from build123d import *

# Parameters (mm, degrees)
SKETCH1_W                 = 60
SKETCH1_H                 = 50
BOSS_EXTRUDE1_DEPTH       = 40
SKETCH2_W                 = 70
SKETCH2_H                 = 70
BOSS_EXTRUDE2_DEPTH       = 1.5
SHELL1_START              = -28
SHELL1_OUTLINE_W          = 46
SHELL1_OUTLINE_H          = 39.5
SHELL1_DEPTH              = 56
F_3_0MM_DOWEL_HOLE2_D     = 3
F_3_0MM_DOWEL_HOLE2_DEPTH = 41.499
FILLET1_R                 = 2
CUT_EXTRUDE2_DEPTH        = 84.200060096
CUT_EXTRUDE2_DEPTH_BACK   = 84.200060096
SKETCH8_W                 = 56
SKETCH8_H                 = 39.5
SKETCH9_W                 = 1.5
SKETCH9_H                 = 70
CUT_EXTRUDE3_DEPTH        = 2


# Read off the part's stored shape, not the designer's step: Shell1
with BuildPart() as part:
    # Sketch1 → Boss-Extrude1 (new body)
    with BuildSketch(Plane.XY):
        Rectangle(SKETCH1_W, SKETCH1_H)
    extrude(amount=BOSS_EXTRUDE1_DEPTH)

    # Sketch2 → Boss-Extrude2 (add)
    with BuildSketch(Plane.XY.offset(40)):
        with Locations((-5, 0)):
            Rectangle(SKETCH2_W, SKETCH2_H)
    extrude(amount=BOSS_EXTRUDE2_DEPTH)

    # Shell1 outline → Shell1 (cut)
    with BuildSketch(Plane.YZ.offset(SHELL1_START)):
        with Locations((0, 21.75)):
            Rectangle(SHELL1_OUTLINE_W, SHELL1_OUTLINE_H)
    extrude(amount=SHELL1_DEPTH, mode=Mode.SUBTRACT)

    # Ø3.0mm Dowel Hole2
    with Locations(Plane(origin=(-311.781139065, -231.688044449, 0), x_dir=(-1, 0, 0), z_dir=(0, 0, -1))):
        with Locations((-327.471139065, 246.969744449), (-297.471139065, 246.969744449), (-297.471139065, 214.569744449), (-327.471139065, 214.569744449)):
            Hole(F_3_0MM_DOWEL_HOLE2_D / 2, depth=F_3_0MM_DOWEL_HOLE2_DEPTH)

    # Fillet1
    fillet1_edges = [part.edges().sort_by_distance(p)[0] for p in [
        (0, -25, 0),
        (-30, 0, 0),
        (0, 25, 0),
        (30, 0, 0),
        (30, -25, 20),
        (-30, -25, 20),
        (-30, 25, 20),
        (30, 25, 20),
    ]]
    fillet(fillet1_edges, radius=FILLET1_R)

    # Sketch8 → Cut-Extrude2 (cut, two sides: drawn at the far end of the back side and taken through both)
    with BuildSketch(Plane.XZ.offset(25).offset(-CUT_EXTRUDE2_DEPTH_BACK)):
        with Locations((0, 21.75)):
            Rectangle(SKETCH8_W, SKETCH8_H)
    extrude(amount=CUT_EXTRUDE2_DEPTH + CUT_EXTRUDE2_DEPTH_BACK, mode=Mode.SUBTRACT)

    # Sketch9 → Cut-Extrude3 (cut)
    with BuildSketch(Plane(origin=(30, 0, 0), x_dir=(0, 0, -1), z_dir=(1, 0, 0))):
        with Locations((-40.75, 0)):
            Rectangle(SKETCH9_W, SKETCH9_H)
    extrude(amount=-CUT_EXTRUDE3_DEPTH, mode=Mode.SUBTRACT)


solid = part.part
CAD build for the part. Positions are in the model's coordinates, mm. A direction names the side the tool comes from. Round coordinates to 2 decimals unless told otherwise and drop trailing zeros. Write each loop counter-clockwise with the first axis right and the second up, starting at its lowest first coordinate (ties: lowest second). Pieces come first, ordered by that corner, then holes.
(1) Slice it at C-C, the plane y = 21. Write the cut outline in (x, z), and give its area (3 significant figures).
(2) Slice it at A-A, the plane x = 15.69. Write the cut outline in (y, z).
(3) Drop flat-ended pins along their axis: P1, Ø3, axis at x = 8.5, y = 12, coming from the -Z side; P2, Ø10, axis at y = 25.5, z = 12.5, coming from the -X side; P3, Ø10, axis at x = -19, z = 5.5, coming from the -Y side; P4, Ø2.5, axis at x = -14.31, y = -17.12, coming from the +Z side. Give the stop position or say it passes through.
(4) Probe line 1 along X through (y, z) = (-6.5, 20.5); line 2 along Y through (x, z) = (15.69, 1.4); line 3 along Z through (x, y) = (-36, 22.5). List the from-to ranges inside material, lowest first.
(5) 3-axis set-ups, long thin cutter, end or side, ignore diameter. For faces 4 (the face through (-29.4, 24.43, 21.27)), 5 (the face through (-30, 0, 21)), 6 (the face through (28, 0, 21)), 7 (the face through (-29.43, -24.4, 21.27)): which of +Z, -Z, +X, -X, +Y, -Y reach the whole face in a straight line?
(6) Slice it at D-D, the plane x = 25.5. Write the cut outline in (y, z).
(7) Mould opens along X. For faces 1 (the face through (-12.88, -16.67, 1.01)), 2 (the face through (29.43, 0.32, 0.6)), 3 (the face through (0.39, 24.43, 0.6)) say: pulls with the +X half, pulls with the -X half, needs draft (parallel to the pull), parting line crosses it, or undercut.
(8) Slice it at B-B, the plane z = 27. Write the cut outline in (x, y), and give its area (3 significant figures).
From the geometry:
1. outline: (-40, 40) - (-30, 40) - (-30, 2) arc R2 ccw to (-28, 0) - (28, 0) arc R2 ccw to (30, 2) - (30, 40) - (28, 40) - (28, 2) - (-28, 2) - (-28, 41.5) - (-40, 41.5) - close
1. area: 288 mm2
2. outline: (-25, 2) arc R2 ccw to (-23, 0) - (-18.62, 0) - (-18.62, 2) - close; (-15.62, 0) - (13.78, 0) - (13.78, 2) - (-15.62, 2) - close; (16.78, 0) - (23, 0) arc R2 ccw to (25, 2) - (16.78, 2) - close
3. P1: stops at z = 0
3. P2: stops at x = -30
3. P3: stops at y = -25
3. P4: passes through
4. line 1: x = -30 to -28, 28 to 30
4. line 2: y = -24.91 to -18.62, -15.62 to 13.78, 16.78 to 24.91
4. line 3: z = 40 to 41.5
5. face 4: -Z, -X, +Y
5. face 5: -Z, -X, +Y, -Y
5. face 6: +Z, +Y, -Y
5. face 7: -Z, -X, -Y
6. outline: (-25, 2) arc R2 ccw to (-23, 0) - (23, 0) arc R2 ccw to (25, 2) - close
7. face 1: undercut
7. face 2: pulls with the +X half
7. face 3: needs draft
8. outline: (-30, -23) arc R2 ccw to (-28, -25) - (-28, 25) arc R2 ccw to (-30, 23) - close; (28, -25) arc R2 ccw to (30, -23) - (30, 23) arc R2 ccw to (28, 25) - close
8. area: 197 mm2
